Autodesk Inventor part; units mm, degrees
ref_plane "YZ Plane" through (0, 0, 0) normal (1, 0, 0) x (0, 1, 0)
ref_plane "XZ Plane" through (0, 0, 0) normal (0, 1, 0) x (-1, 0, 0)
ref_plane "XY Plane" through (0, 0, 0) normal (0, 0, 1) x (1, 0, 0)
sketch "Sketch1" plane through (0, 0, 0) normal (0, 1, 0) x (-1, 0, 0)
  line L0 (-78, 0) -> (-78, -60)
  line L1 (-78, -60) -> (0, -60)
  line L2 (0, -60) -> (0, 0)
  arc A0 (-43, 0) -> (-35, 0) centre (-39, 0) ccw
  circle A1 centre (-39, -30) radius 12
  line L3 (-23.5, -14.5) -> (-54.5, -14.5)
  circle A2 centre (-23.5, -45.5) radius 1.5
  circle A3 centre (-54.5, -45.5) radius 1.5
  circle A4 centre (-54.5, -14.5) radius 1.5
  circle A5 centre (-23.5, -14.5) radius 1.5
  line L4 (0, 0) -> (-35, 0)
  line L5 (-43, 0) -> (-78, 0)
  dimension "d1" = 60
  dimension "d2" = 78
  dimension "d3" = 8
  dimension "d5" = 24
  dimension "d15" = 31
  dimension "d16" = 3
  dimension "d17" = 3
  dimension "d18" = 3
  dimension "d19" = 3
extrude "Extrusion1" add sketch "Sketch1" along normal blind 20
sketch "Sketch2" plane through (78, 0, -60) normal (0, 0, -1) x (-1, 0, 0)
  circle A0 centre (10, 10) radius 4
  circle A1 centre (68, 10) radius 4
  dimension "d24" = 8
  dimension "d25" = 8
extrude "Extrusion2" cut sketch "Sketch2" against normal blind 100
sketch "Sketch3" plane through (0, 20, 0) normal (0, 1, 0) x (1, 0, 0)
  circle A0 centre (39, 30) radius 12
  circle A1 centre (23.5, 14.5) radius 1.5
  circle A2 centre (54.5, 14.5) radius 1.5
  circle A3 centre (54.5, 45.5) radius 1.5
  circle A4 centre (23.5, 45.5) radius 1.5
  line L0 (60.5, 8.5) -> (17.5, 8.5)
  line L1 (17.5, 8.5) -> (17.5, 51.5)
  line L2 (17.5, 51.5) -> (60.5, 51.5)
  line L3 (60.5, 51.5) -> (60.5, 8.5)
  line L4 (60.5, 8.5) -> (17.5, 51.5) construction
  line L5 (17.5, 8.5) -> (60.5, 51.5) construction
  dimension "d28" = 43
  dimension "d29" = 43
extrude "Extrusion3" cut sketch "Sketch3" against normal blind 5
properties part number "Z_MotorMount_RodHolder_V2" material "Birch"
Can you work these out from the model? Positions are in its coordinate system, mm. A direction names the side the tool comes from. Give positions to 0.01 mm unless a question says otherwise; leave off trailing zeros. Loops run counter-clockwise (first coordinate to the right, second up) from the corner with the lowest first, then second, coordinate; pieces in that order, holes last. Notation, with made-up numbers: M -16.75,47.25 L 24.25,47.25 A34 cw 24.25,80.25 Z; hole C 22,65 d9. An arc over 180 degrees is marked long. Use one line per item in the form item = value. Start each with the question number.
(1) I'm going to push flat-ended pins straight in: P1, Ø4, axis at x = 47, z = -38, coming from the +Y side; P2, Ø2.5, axis at x = 54.5, z = -14.5, coming from the +Y side. Where does each tip first touch, or does it pass through?
(2) I want a section at D-D, the plane z = -30. Write out the boundary of the cut face in (x, y).
(3) I want a section at A-A, the plane z = -45.5. Write out the boundary of the cut face in (x, y).
(4) I want a section at B-B, the plane x = 23.5. Write out the boundary of the cut face in (y, z).
(5) On a 3-axis mill with a long thin cutter (end or side, diameter ignored), from which of +Z, -Z, +X, -X, +Y, -Y can I reach the whole of each face in a straight line? I mean faces 1 (the flat face through (39, 18, -8.5)), 2 (the flat face through (66, 20, -30)). Say none if no direction works.
(6) Thinking about a two-plate mould opening in X: for faces 3 (the flat face through (0, 10, -30)), 4 (the cylindrical face through (39, 10, -4)), 5 (the flat face through (40, 10, -60)), which applies, released by +X, released by -X, zero draft, split by the parting line, or undercut?
(7) Please list where these lines run through material, in increasing order: line 1 (Z direction, x = 54.5, y = 3); line 2 (X direction, y = 4.5, z = -45); line 3 (Y direction, x = 10, z = -28.5).
(8) I want a section at C-C, the plane y = 10. Write out the boundary of the cut face in (x, z), and give its area (3 significant figures).
Worked out:
q1.P1 = 15
q1.P2 = through
q2.outline = M 0,0 L 27,0 L 27,15 L 17.5,15 L 17.5,20 L 0,20 Z; M 51,0 L 78,0 L 78,20 L 60.5,20 L 60.5,15 L 51,15 Z; hole C 10,10 d8; hole C 68,10 d8
q3.outline = M 0,0 L 22,0 L 22,15 L 17.5,15 L 17.5,20 L 0,20 Z; M 25,0 L 53,0 L 53,15 L 25,15 Z; M 56,0 L 78,0 L 78,20 L 60.5,20 L 60.5,15 L 56,15 Z; hole C 10,10 d8; hole C 68,10 d8
q4.outline = M 0,-60 L 20,-60 L 20,-51.5 L 15,-51.5 L 15,-47 L 0,-47 Z; M 0,-44 L 15,-44 L 15,-16 L 0,-16 Z; M 0,-13 L 15,-13 L 15,-8.5 L 20,-8.5 L 20,0 L 0,0 Z
q5.face_1 = +Y
q5.face_2 = +Z, -Z, +X, -X, +Y
q6.face_3 = released by -X
q6.face_4 = undercut
q6.face_5 = zero draft
q7.line_1 = -60 to -47, -44 to -16, -13 to 0
q7.line_2 = 0 to 22.09, 24.91 to 53.09, 55.91 to 78
q7.line_3 = 0 to 6, 14 to 20
q8.outline = M 0,-60 L 6,-60 L 6,0 L 0,0 Z; M 14,-60 L 64,-60 L 64,0 L 43,0 A4 cw 35,0 L 14,0 Z; M 72,-60 L 78,-60 L 78,0 L 72,0 Z; hole C 23.5,-45.5 d3; hole C 23.5,-14.5 d3; hole C 39,-30 d24; hole C 54.5,-45.5 d3; hole C 54.5,-14.5 d3
q8.area = 3,210 mm²
